Model file for the job. Use its own axes, mm. Coordinates: 2 decimals unless noted, no trailing zeros. Loops run counter-clockwise (first coordinate to the right, second up) from the corner with the lowest first, then second, coordinate; pieces in that order, holes last.
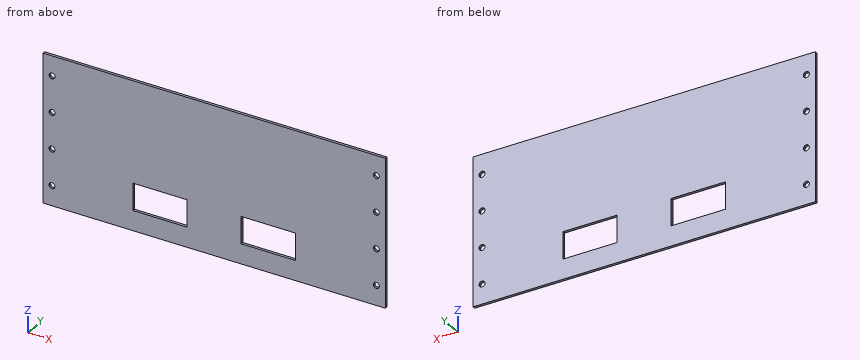
from build123d import *

# Parameters (mm, degrees)
SKETCH_W       = 190
SKETCH_H       = 82
SKETCH_R       = 1.65
PAD_DEPTH      = 0.75
PAD_DEPTH_BACK = 0.75
SKETCH001_W    = 30
SKETCH001_H    = 15
POCKET_DEPTH   = 5


with BuildPart() as part:
    # Sketch → Pad (new body, two sides)
    with BuildSketch(Plane.XZ) as pad_sk:
        Rectangle(SKETCH_W, SKETCH_H)
        with Locations((90, 30)):
            Circle(SKETCH_R, mode=Mode.SUBTRACT)
        with Locations((90, 10)):
            Circle(SKETCH_R, mode=Mode.SUBTRACT)
        with Locations((90, -30)):
            Circle(SKETCH_R, mode=Mode.SUBTRACT)
        with Locations((90, -10)):
            Circle(SKETCH_R, mode=Mode.SUBTRACT)
        with Locations((-90, 30)):
            Circle(SKETCH_R, mode=Mode.SUBTRACT)
        with Locations((-90, 10)):
            Circle(SKETCH_R, mode=Mode.SUBTRACT)
        with Locations((-90, -30)):
            Circle(SKETCH_R, mode=Mode.SUBTRACT)
        with Locations((-90, -10)):
            Circle(SKETCH_R, mode=Mode.SUBTRACT)
    extrude(amount=PAD_DEPTH)
    extrude(pad_sk.sketch, amount=-PAD_DEPTH_BACK)

    # Sketch001 (on Face14 of Pad) → Pocket (cut)
    with BuildSketch(Plane.XZ.offset(0.75)):
        with Locations((-30, -22.5)):
            Rectangle(SKETCH001_W, SKETCH001_H)
        with Locations((30, -22.5)):
            Rectangle(SKETCH001_W, SKETCH001_H)
    extrude(amount=-POCKET_DEPTH, mode=Mode.SUBTRACT)


solid = part.part
Q1. Slice it at A-A (x = -19). List the corners of the cut face in (y, z).
Answers:
outline: (-0.75, -41) - (0.75, -41) - (0.75, -30) - (-0.75, -30) - close; (-0.75, -15) - (0.75, -15) - (0.75, 41) - (-0.75, 41) - close
Q2. Drill centre lines: line 1 (Z direction, x = -90, y = -0.35); line 2 (X direction, y = 0.05, z = -20); line 3 (Z direction, x = -31.5, y = 0.2). Where is each one in solid material? Low to high.
Answers:
line 1: z = -41 to -31.65, -28.35 to -11.65, -8.35 to 8.35, 11.65 to 28.35, 31.65 to 41
line 2: x = -95 to -45, -15 to 15, 45 to 95
line 3: z = -41 to -30, -15 to 41
Q3. Slice it at B-B (y = -0.5). Count the separate pieces of the cut face and the enclosed holes in it, and give its area (3 significant figures).
Answers:
separate pieces: 1
enclosed holes: 10
area: 14,600 mm2
